The model under review builds one solid part; all positions refer to its coordinate system, in mm. Face numbers are marked on the shaded views. A direction names the side the tool comes from. Give positions to 0.01 mm unless a question says otherwise; leave off trailing zeros. Loops run counter-clockwise (first coordinate to the right, second up) from the corner with the lowest first, then second, coordinate; pieces in that order, holes last. Notation, with made-up numbers: (43, 37.25) - (66, 37.25) arc R19 cw to (66, 57.25) - close; hole circle Ø2 at (78.5, -22.75). An arc over 180 degrees is marked (long way). Return JSON: item names as keys, results as strings. Group by question number.
```python
from build123d import *

# Parameters (mm, degrees)
F0_W      = 80
F0_H      = 58
F1_DEPTH  = 50
F3_DEPTH  = 80.001
F6_DEPTH  = 40
F7_W      = 8
F7_H      = 20
F8_DEPTH  = 15
F10_DEPTH = 40.001


with BuildPart() as f1:
    # F0 (on Top) → F1 (new body)
    with BuildSketch(Plane.XY):
        Rectangle(F0_W, F0_H)
    extrude(amount=F1_DEPTH)

    # F2 (on face) → F3 (cut, through all)
    with BuildSketch(Plane(origin=(-40, 0, 0), x_dir=(0, -1, 0), z_dir=(-1, 0, 0))):
        Polygon((29, 50), (11, 50), (11, 23.0452120304), (21, 23.0452120304), (29, 0), align=None)
    extrude(amount=-F3_DEPTH, mode=Mode.SUBTRACT)

    # F5 (on offset) → F6 (cut)
    with BuildSketch(Plane(origin=(-20, 0, 0), x_dir=(0, -1, 0), z_dir=(-1, 0, 0))):
        Polygon((24.8185806181, 12.0452120304), (21, 23.0452120304), (16, 23.0452120304), (16, 12.0452120304), align=None)
    extrude(amount=-F6_DEPTH, mode=Mode.SUBTRACT)

    # F7 (on face) → F8 (cut)
    with BuildSketch(Plane.XY.offset(50)):
        with Locations((-28, 9)):
            Rectangle(F7_W, F7_H)
        with Locations((28, 9)):
            Rectangle(F7_W, F7_H)
    extrude(amount=-F8_DEPTH, mode=Mode.SUBTRACT)

    # F9 (on face) → F10 (cut, through all)
    with BuildSketch(Plane.XZ.offset(11)):
        with BuildLine():
            Line((25, 50), (-25, 50))
            ThreePointArc((-25, 50), (0, 25), (25, 50))
        make_face()
    extrude(amount=-F10_DEPTH, mode=Mode.SUBTRACT)


solid = f1.part
```
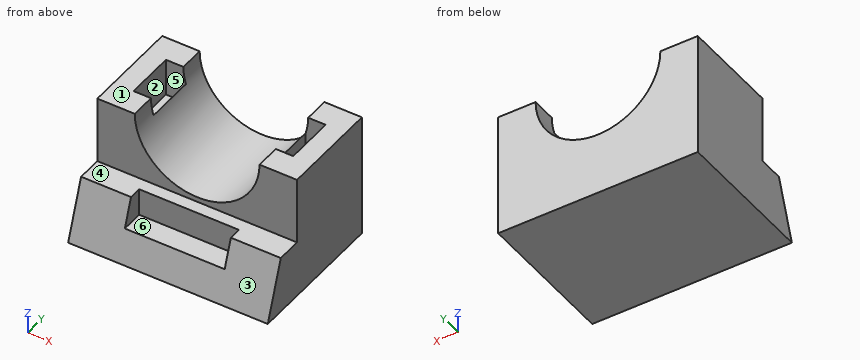
1) We need section D-D, the plane y = -2. Write out the cut boundary in (x, z), plus the area to 3 significant figures.
2) We need section C-C, the plane z = 45.5. Write out the cut boundary in (x, y), plus the area to 3 significant figures.
3) We need section A-A, the plane z = 37. Write out the cut boundary in (x, y), plus the area to 3 significant figures.
4) We need section B-B, the plane x = 0. Write out the cut boundary in (y, z).
5) For pin 1 Ø5 at (x, z) = (-7, 13) entering from -Y (3 decimals); pin 2 Ø6.5 at (x, z) = (29, 40.5) entering from -Y; pin 3 Ø10 at (x, y) = (-6.5, -12) entering from +Z, all flat-tipped, find the tip position at first contact; note any pin that passes through.
6) Draft analysis for pull direction Y (two halves, no side actions). For the marked faces 1, 2 and 3, state which applies: +Y half, -Y half, draft (parallel to the pull), parting line (faces both ways), or undercut.
7) Tool access review of the marked faces 4, 5 and 6: name each direction out of +Z, -Z, +X, -X, +Y, -Y from which nothing blocks a thin tool from reaching the whole face with its end or side.
8) To check wall thickness, follow line 1 (X direction, y = 5, z = 38); line 2 (Z direction, x = -0.5, y = -14); line 3 (Z direction, x = 0, y = 2.5). State the ranges of each line that lie inside material, in increasing order.
Findings:
{
 "1": {"outline": "(-40, 0) - (40, 0) - (40, 50) - (25, 50) arc R25 cw to (-25, 50) - (-40, 50) - close", "area": "3,020 mm^2"},
 "2": {"outline": "(-40, -11) - (-24.59, -11) - (-24.59, -1) - (-32, -1) - (-32, 19) - (-24.59, 19) - (-24.59, 29) - (-40, 29) - close; (24.59, -11) - (40, -11) - (40, 29) - (24.59, 29) - (24.59, 19) - (32, 19) - (32, -1) - (24.59, -1) - close", "area": "936 mm^2"},
 "3": {"outline": "(-40, -11) - (-21.35, -11) - (-21.35, 29) - (-40, 29) - close; (21.35, -11) - (40, -11) - (40, 29) - (21.35, 29) - close; hole (-32, -1) - (-24, -1) - (-24, 19) - (-32, 19) - close; hole (24, -1) - (32, -1) - (32, 19) - (24, 19) - close", "area": "1,170 mm^2"},
 "4": {"outline": "(-29, 0) - (29, 0) - (29, 25) - (-11, 25) - (-11, 23.05) - (-16, 23.05) - (-16, 12.05) - (-24.82, 12.05) - close"},
 "5": {"pin 1": "stops at y = -25.355", "pin 2": "stops at y = -11", "pin 3": "stops at z = 27.75"},
 "6": {"face 1": "draft", "face 2": "undercut", "face 3": "-Y half"},
 "7": {"face 4": "+Z, +X, -X, -Y", "face 5": "+Z", "face 6": "+Z, -Y"},
 "8": {"line 1": "x = -40 to -32, -24 to -21.93, 21.93 to 24, 32 to 40", "line 2": "z = 0 to 23.05", "line 3": "z = 0 to 25"}
}
